from build123d import *

# Parameters (mm, degrees)
F0_W     = 70
F0_H     = 70
F0_W_2   = 56
F0_H_2   = 56
F1_DEPTH = 55
F2_DEPTH = 380
F3_R     = 20
F4_DEPTH = 70.001


with BuildPart() as f1:
    # F0 (on Front) → F1 (new body)
    with BuildSketch(Plane.XZ):
        Rectangle(F0_W, F0_H)
        Rectangle(F0_W_2, F0_H_2, mode=Mode.SUBTRACT)
    extrude(amount=F1_DEPTH)

    # F0 (on Front) → F2 (join)
    with BuildSketch(Plane.XZ):
        Rectangle(F0_W, F0_H)
        Rectangle(F0_W_2, F0_H_2, mode=Mode.SUBTRACT)
        Rectangle(F0_W_2, F0_H_2)
    extrude(amount=-F2_DEPTH)

    # F3 (on face) → F4 (cut, through all)
    with BuildSketch(Plane.YZ.offset(35)):
        with BuildLine():
            ThreePointArc((124, 30), (145.2132034356, 21.2132034356), (154, 0))
            ThreePointArc((154, 0), (145.2132034356, -21.2132034356), (124, -30))
            add(Edge.make_bspline(
                [(124, -30), (103.2983378934, -30), (72.7074229784, -29.9876599501), (43.9366263473, -30.7832092477), (36.1074860936, -35), (-10, -35)],
                knots=[0, 0, 0, 0, 0.3730126835, 0.6041485586, 1, 1, 1, 1], degree=3))
            Line((-10, -35), (380, -35))
            Line((380, -35), (380, 35))
            Line((380, 35), (-10, 35))
            add(Edge.make_bspline(
                [(124, 30), (103.2983378934, 30), (72.7074229784, 29.9876599501), (43.9366263473, 30.7832092477), (36.1074860936, 35), (-10, 35)],
                knots=[0, 0, 0, 0, 0.3730126835, 0.6041485586, 1, 1, 1, 1], degree=3))
        make_face()
        with Locations((124, 0)):
            Circle(F3_R)
    extrude(amount=-F4_DEPTH, mode=Mode.SUBTRACT)


solid = f1.part
Here's how the part is built. I have some questions about the finished solid (model axes, mm). A direction names the side the tool comes from. Round coordinates to 2 decimals unless told otherwise and drop trailing zeros. Order: outer loops, then holes, each group sorted by start corner. A loop starts at its lowest first (then second) coordinate and runs counter-clockwise, first axis right, second up. Notation, with made-up numbers: M 28.5,80 L 56.5,80 A25 ccw 56.5,106 Z; hole C -35.75,-32.75 d11. An arc over 180 degrees is marked long. Return JSON: item names as keys, results as strings. Group by question number.
1. If we mould it in two halves opening along Z, with no side actions, what happens to faces 1 (the face through (0.49, 153.993, 0.66)), 2 (the face through (-32, -55, 0)), 3 (the face through (28, -27, 0)), 4 (the face through (0, -33, -35))? For each: pulls with the +Z half, pulls with the -Z half, needs draft (parallel to the pull), parting line crosses it, or undercut.
2. If we section it at A-A on z = 0: List the corners of the cut face in (x, y) for me, then the cut area to 3 significant figures.
3. If we section it at B-B on y = -31: List the corners of the cut face in (x, z) for me, then the cut area to 3 significant figures.
4. On a 3-axis mill with a long thin cutter (end or side, diameter ignored), from which of +Z, -Z, +X, -X, +Y, -Y can I reach the whole of each face in a straight line? I mean faces 5 (the face through (0, -33, 35)), 6 (the face through (-28, -27, 0)). Say none if no direction works.
5. If we section it at C-C on y = 134: List the corners of the cut face in (x, z) for me.
6. I'm going to push flat-ended pins straight in: pin 1 Ø8 at (x, y) = (-4.5, 54) entering from -Z; pin 2 Ø5 at (x, z) = (-7.5, 5.5) entering from -Y; pin 3 Ø4 at (x, z) = (27.5, 16.5) entering from +Y. Where does each tip first touch, or does it pass through?
7. If we section it at D-D on z = -16: List the corners of the cut face in (x, y) for me, then the cut area to 3 significant figures.
8. Please list where these lines run through material, in increasing order: probe 1 along Y at (x, z) = (30.5, 1); probe 2 along X at (y, z) = (-18.5, 8.5); probe 3 along Z at (x, y) = (-11, 124).
Reply:
{
 "1": {"face 1": "parting line crosses it", "face 2": "needs draft", "face 3": "undercut", "face 4": "pulls with the -Z half"},
 "2": {"outline": "M -35,-55 L -28,-55 L -28,0 L 28,0 L 28,-55 L 35,-55 L 35,104 L -35,104 Z; M -35,144 L 35,144 L 35,154 L -35,154 Z", "area": "8,750 mm^2"},
 "3": {"outline": "M -35,-35 L 35,-35 L 35,35 L -35,35 Z; hole M -28,-28 L 28,-28 L 28,28 L -28,28 Z", "area": "1,760 mm^2"},
 "4": {"face 5": "+Z, +X, -X, +Y, -Y", "face 6": "-Y"},
 "5": {"outline": "M -35,-28.28 L 35,-28.28 L 35,-17.32 L -35,-17.32 Z; M -35,17.32 L 35,17.32 L 35,28.28 L -35,28.28 Z"},
 "6": {"pin 1": "z = -31.17", "pin 2": "y = 0", "pin 3": "y = 150.26"},
 "7": {"outline": "M -35,-55 L -28,-55 L -28,0 L 28,0 L 28,-55 L 35,-55 L 35,112 L -35,112 Z; M -35,136 L 35,136 L 35,149.38 L -35,149.38 Z", "area": "9,550 mm^2"},
 "8": {"probe 1": "-55 to 104.03, 143.97 to 153.98", "probe 2": "-35 to -28, 28 to 35", "probe 3": "-30 to -20, 20 to 30"}
}
